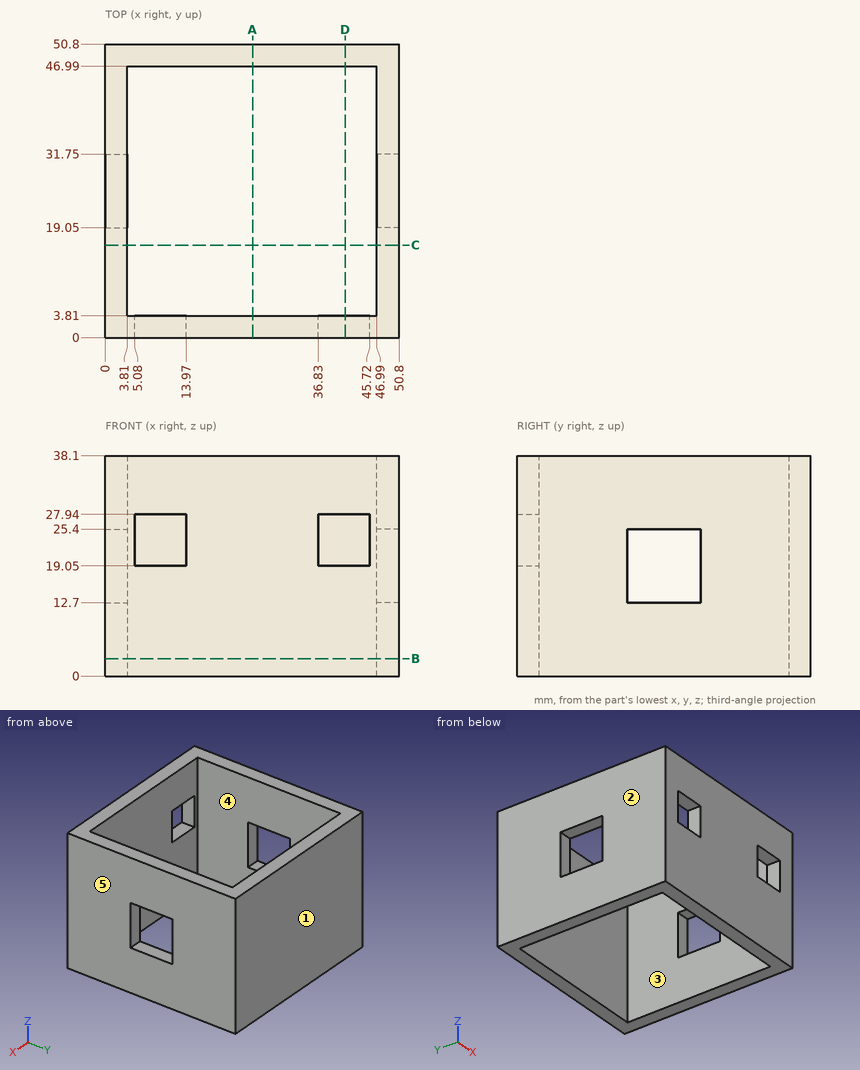
Print and shaded views of the part. All mm, measured from the part's lowest x, y and z. A direction names the side the tool comes from. Round coordinates to 2 decimals unless told otherwise and drop trailing zeros. Write each loop counter-clockwise with the first axis right and the second up, starting at its lowest first coordinate (ties: lowest second). Pieces come first, ordered by that corner, then holes.
(1) Slice it at A-A, the plane x = 25.5. Write the cut outline in (y, z).
(2) Probe line 1 along X through (y, z) = (8, 31); line 2 along Y through (x, z) = (49, 14). List the from-to ranges inside material, lowest first.
(3) 3-axis set-ups, long thin cutter, end or side, ignore diameter. For the marked faces 4 and 5: which of +Z, -Z, +X, -X, +Y, -Y reach the whole face in a straight line?
(4) Mould opens along X. For the marked faces 1, 2 and 3 say: pulls with the +X half, pulls with the -X half, needs draft (parallel to the pull), parting line crosses it, or undercut.
(5) Slice it at D-D, the plane x = 41.5. Write the cut outline in (y, z), and give its area (3 significant figures).
(6) Slice it at B-B, the plane z = 3. Write the cut outline in (x, y), and give its area (3 significant figures).
From the geometry:
1. outline: (0, 0) - (3.81, 0) - (3.81, 38.1) - (0, 38.1) - close; (46.99, 0) - (50.8, 0) - (50.8, 38.1) - (46.99, 38.1) - close
2. line 1: x = 0 to 3.81, 46.99 to 50.8
2. line 2: y = 0 to 19.05, 31.75 to 50.8
3. face 4: +Z, -Z
3. face 5: +Z, -Z, +X, +Y, -Y
4. face 1: needs draft
4. face 2: pulls with the -X half
4. face 3: undercut
5. outline: (0, 0) - (3.81, 0) - (3.81, 19.05) - (0, 19.05) - close; (0, 27.94) - (3.81, 27.94) - (3.81, 38.1) - (0, 38.1) - close; (46.99, 0) - (50.8, 0) - (50.8, 38.1) - (46.99, 38.1) - close
5. area: 256 mm2
6. outline: (0, 0) - (50.8, 0) - (50.8, 50.8) - (0, 50.8) - close; hole (3.81, 3.81) - (46.99, 3.81) - (46.99, 46.99) - (3.81, 46.99) - close
6. area: 716 mm2
